Design review of the part shown in the three views and the two pictorial views. Dimensions are in mm from the part's minimum x, y and z. Give positions to 0.01 mm unless a question says otherwise; leave off trailing zeros. Loops run counter-clockwise (first coordinate to the right, second up) from the corner with the lowest first, then second, coordinate; pieces in that order, holes last. Notation, with made-up numbers: (-2.5, 58) -> (21.5, 58) arc R29 ccw to (21.5, 93) -> close; hole circle Ø5 at (49, 47). An arc over 180 degrees is marked (long way). Answer as CSV lines item,"result".
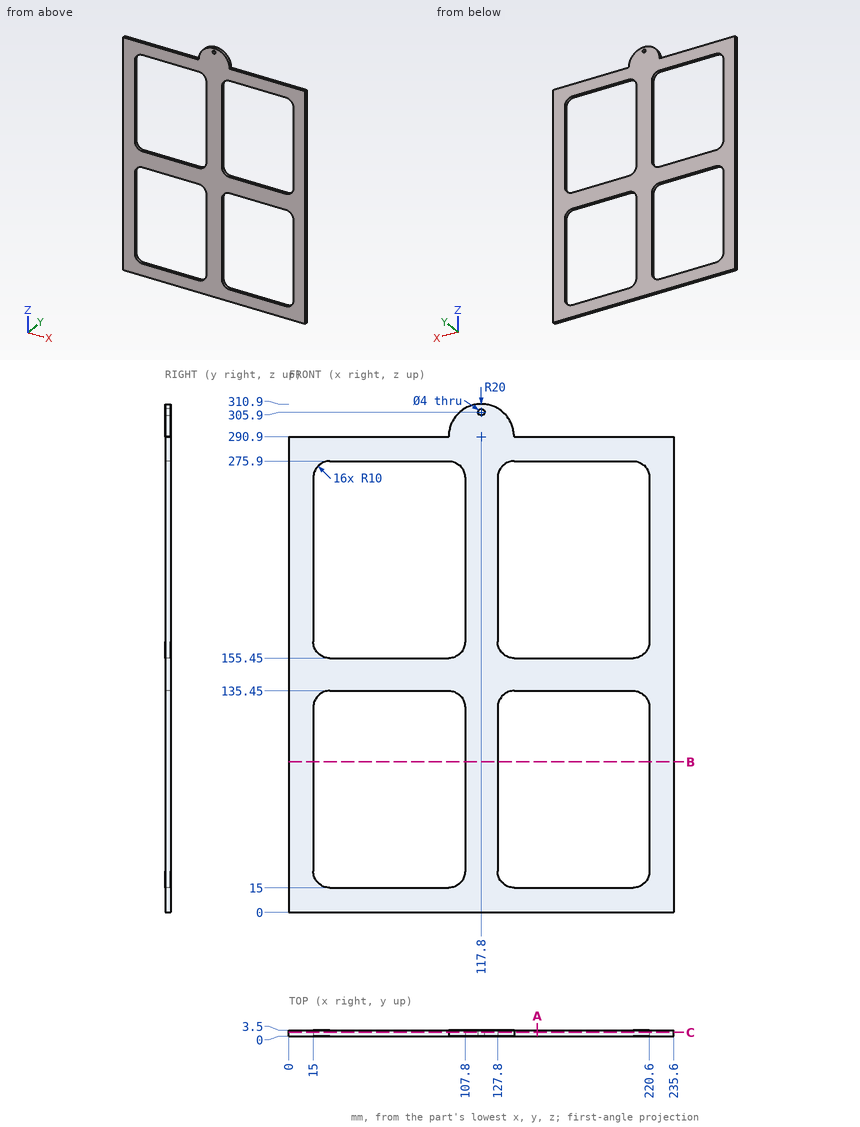
Q1. Clearance check with a flat-ended pin moving along its axis: pin 1 Ø1 at (x, y) = (194, 1.5) entering from +Z. State where the tip first meets the part, or that it passes through.
Filled sheet:
pin 1,"stops at z = 290.9"
Q2. We need section A-A, the plane x = 152. State the section outline as (y, z) points.
Filled sheet:
outline,"(0, 0) -> (3.5, 0) -> (3.5, 15) -> (0, 15) -> close; (0, 135.45) -> (3.5, 135.45) -> (3.5, 155.45) -> (0, 155.45) -> close; (0, 275.9) -> (3.5, 275.9) -> (3.5, 290.9) -> (0, 290.9) -> close"
Q3. We need section B-B, the plane z = 92. State the section outline as (x, y) points, and give its area (3 significant figures).
Filled sheet:
outline,"(0, 0) -> (15, 0) -> (15, 3.5) -> (0, 3.5) -> close; (107.8, 0) -> (127.8, 0) -> (127.8, 3.5) -> (107.8, 3.5) -> close; (220.6, 0) -> (235.6, 0) -> (235.6, 3.5) -> (220.6, 3.5) -> close"
area,"175 mm^2"
Q4. To check wall thickness, follow probe 1 along X at (y, z) = (3.05, 98.5); probe 2 along Z at (x, y) = (80, 2.2); probe 3 along X at (y, z) = (1.8, 132). State the ranges of each line that lie inside material, in increasing order. Write a range as from..to.
Filled sheet:
probe 1,"x = 0..15, 107.8..127.8, 220.6..235.6"
probe 2,"z = 0..15, 135.45..155.45, 275.9..290.9"
probe 3,"x = 0..17.44, 105.36..130.24, 218.16..235.6"
Q5. We need section C-C, the plane y = 2.2. State how many separate pieces and enclosed holes the cut face has, and give its area (3 significant figures).
Filled sheet:
separate pieces,"1"
enclosed holes,"5"
area,"24,800 mm^2"
